```python
from build123d import *

# Parameters (mm, degrees)
SKETCH2_W           = 63.5
SKETCH2_H           = 88.5
BOSS_EXTRUDE1_DEPTH = 2
SKETCH3_W           = 63.5
SKETCH3_H           = 88.5
SKETCH3_W_2         = 59.5
SKETCH3_H_2         = 84.5
BOSS_EXTRUDE2_DEPTH = 20
SKETCH4_W           = 6.35
SKETCH4_H           = 13
SKETCH4_H_2         = 10.9
CUT_EXTRUDE1_DEPTH  = 2
CHAMFER1_SIZE       = 0.5
SKETCH5_R           = 0.75
SKETCH5_W           = 6.35
SKETCH5_H           = 25
CUT_EXTRUDE3_DEPTH  = 2
FILLET1_R           = 6


with BuildPart() as part:
    # Sketch2 → Boss-Extrude1 (new body)
    with BuildSketch(Plane.XY.offset(2)):
        with Locations((-8.071244, 16.046786)):
            Rectangle(SKETCH2_W, SKETCH2_H)
    extrude(amount=BOSS_EXTRUDE1_DEPTH)

    # Sketch3 → Boss-Extrude2 (add)
    with BuildSketch(Plane(origin=(0, 0, 2), x_dir=(-1, 0, 0), z_dir=(0, 0, -1))):
        with Locations((8.071244, 16.046786)):
            Rectangle(SKETCH3_W, SKETCH3_H)
        with Locations((8.071244, 16.046786)):
            Rectangle(SKETCH3_W_2, SKETCH3_H_2, mode=Mode.SUBTRACT)
    extrude(amount=BOSS_EXTRUDE2_DEPTH)

    # Sketch4 → Cut-Extrude1 (cut)
    with BuildSketch(Plane(origin=(23.678756, 0, 0), x_dir=(0, 0, -1), z_dir=(1, 0, 0))):
        with Locations((14.825, 35.546786)):
            Rectangle(SKETCH4_W, SKETCH4_H)
        with Locations((14.825, 49.296786)):
            Rectangle(SKETCH4_W, SKETCH4_H_2)
    extrude(amount=-CUT_EXTRUDE1_DEPTH, mode=Mode.SUBTRACT)

    # Chamfer1
    chamfer1_edges = [part.edges().sort_by_distance(p)[0] for p in [
        (23.678756, 42.046786, -14.825),
        (23.678756, 35.546786, -11.65),
        (23.678756, 29.046786, -14.825),
        (23.678756, 54.746786, -14.825),
        (23.678756, 49.296786, -11.65),
        (23.678756, 43.846786, -14.825),
    ]]
    chamfer(chamfer1_edges, length=CHAMFER1_SIZE)

    # Sketch5 → Cut-Extrude3 (cut)
    with BuildSketch(Plane.ZY.offset(39.821244)):
        with Locations(Location((-12.431991388, 40.654286, 0), (0, 0, 270))):
            Circle(SKETCH5_R)
        with Locations((-14.825, 21.706977335)):
            Rectangle(SKETCH5_W, SKETCH5_H)
    extrude(amount=-CUT_EXTRUDE3_DEPTH, mode=Mode.SUBTRACT)

    # Fillet1
    fillet1_edges = [part.edges().sort_by_distance(p)[0] for p in [
        (-38.821244, 34.206977335, -18),
        (-38.821244, 9.206977335, -18),
    ]]
    fillet(fillet1_edges, radius=FILLET1_R)


solid = part.part
```
Part model, mm, in its own coordinate system. A direction names the side the tool comes from. Give positions to 0.01 mm unless a question says otherwise; leave off trailing zeros. Order: outer loops, then holes, each group sorted by start corner. A loop starts at its lowest first (then second) coordinate and runs counter-clockwise, first axis right, second up. Notation, with made-up numbers: M 21,-37 L 29,-37 A22 ccw 29,-28 Z; hole C 44.25,48 d5. An arc over 180 degrees is marked long. Use a Markdown table: item, result. Add a question column.
(1) Saw through at A-A, the plane y = -21. Give the cut face in (x, z), and give its area (3 significant figures).
(2) Drop flat-ended pins along their axis: P1, Ø12, axis at x = -31, y = 32, coming from the -Z side; P2, Ø6, axis at y = 18.5, z = -13, coming from the -X side; P3, Ø2, axis at y = 40.65, z = -12.43, coming from the +X side; P4, Ø0.8, axis at x = 23, y = 33, coming from the -Z side. Give the stop position or say it passes through.
(3) Saw through at B-B, the plane z = -8. Give the cut face in (x, y), and give its area (3 significant figures).
(4) Probe line 1 along X through (y, z) = (-6.5, -2.25); line 2 along Y through (x, z) = (10, -14); line 3 along Z through (x, y) = (-7.5, 52). List the from-to ranges inside material, lowest first. Write a range as [from, to].
(5) Saw through at C-C, the plane x = 14. Give the cut face in (y, z).
(6) Mould opens along X. For faces 1 (the face through (-8, -26.203, -8)), 2 (the face through (23, 43, -18)), 3 (the face through (23.679, 15, -7)) say: +X half, -X half, draft (parallel to the pull), parting line (faces both ways), or undercut.
(7) 3-axis set-ups, long thin cutter, end or side, ignore diameter. For faces 4 (the face through (-38.81, 36.01, -16.29)), 5 (the face through (-8, 60.297, -7)), 6 (the face through (-38.81, 7.4, -16.29)), 7 (the face through (-9, 17, 4)), 8 (the face through (-37.821, 15, -8)): which of +Z, -Z, +X, -X, +Y, -Y reach the whole face in a straight line?
(8) Saw through at D-D, the plane z = -16. Give the cut face in (x, y), and give its area (3 significant figures).
Answer key:
| question | item | result |
|---|---|---|
| 1 | outline | M -39.82,-18 L -37.82,-18 L -37.82,2 L 21.68,2 L 21.68,-18 L 23.68,-18 L 23.68,4 L -39.82,4 Z |
| 1 | area | 207 mm^2 |
| 2 | P1 | z = 2 |
| 2 | P2 | x = -39.82 |
| 2 | P3 | x = 23.4 |
| 2 | P4 | z = -11.65 |
| 3 | outline | M -39.82,-28.2 L 23.68,-28.2 L 23.68,60.3 L -39.82,60.3 Z; hole M -37.82,-26.2 L 21.68,-26.2 L 21.68,58.3 L -37.82,58.3 Z |
| 3 | area | 592 mm^2 |
| 4 | line 1 | [-39.82, -37.82], [21.68, 23.68] |
| 4 | line 2 | [-28.2, -26.2], [58.3, 60.3] |
| 4 | line 3 | [2, 4] |
| 5 | outline | M -28.2,-18 L -26.2,-18 L -26.2,2 L 58.3,2 L 58.3,-18 L 60.3,-18 L 60.3,4 L -28.2,4 Z |
| 6 | face 1 | undercut |
| 6 | face 2 | draft |
| 6 | face 3 | +X half |
| 7 | face 4 | -Z, +X, -X |
| 7 | face 5 | +Z, -Z, +X, -X, +Y |
| 7 | face 6 | -Z, -X |
| 7 | face 7 | +Z, +X, -X, +Y, -Y |
| 7 | face 8 | -Z |
| 8 | outline | M -39.82,-28.2 L 23.68,-28.2 L 23.68,28.55 L 23.18,29.05 L 21.68,29.05 L 21.68,-26.2 L -37.82,-26.2 L -37.82,7.68 L -39.82,7.68 Z; M -39.82,35.73 L -37.82,35.73 L -37.82,58.3 L 21.68,58.3 L 21.68,54.75 L 23.18,54.75 L 23.68,55.25 L 23.68,60.3 L -39.82,60.3 Z; M 21.68,42.05 L 23.18,42.05 L 23.68,42.55 L 23.68,43.35 L 23.18,43.85 L 21.68,43.85 Z |
| 8 | area | 488 mm^2 |
